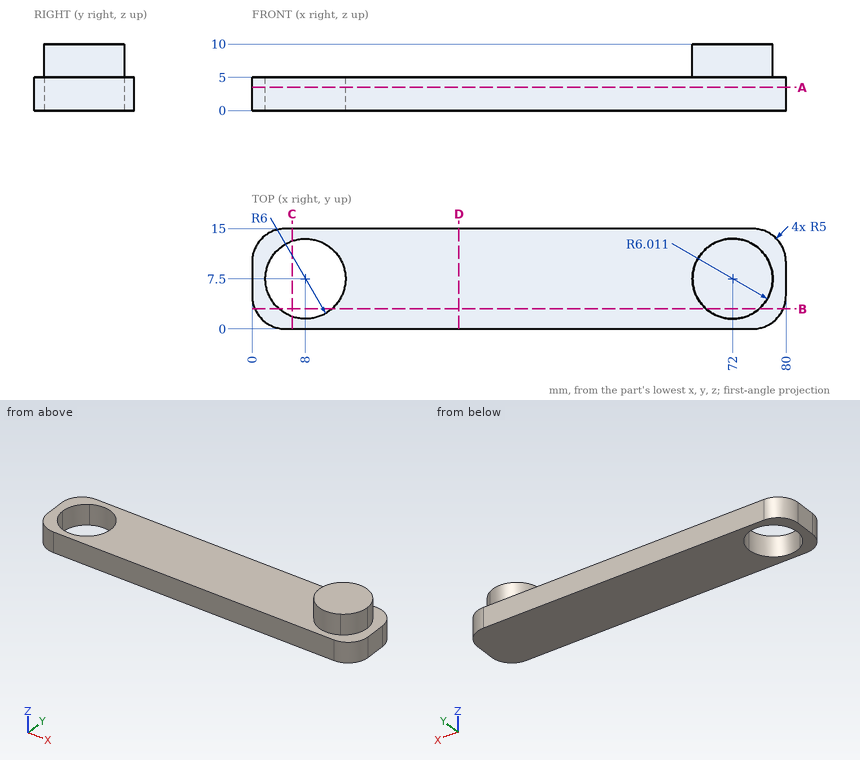
Study the drawing (mm; zero at the part's minimum x, y, z) and answer. Round coordinates to 2 decimals unless told otherwise and drop trailing zeros. Order: outer loops, then holes, each group sorted by start corner. A loop starts at its lowest first (then second) coordinate and runs counter-clockwise, first axis right, second up. Notation, with made-up numbers: (-34.75, 16) -> (-12.75, 16) arc R31 ccw to (-12.75, 45) -> close; hole circle Ø5 at (50.25, 73). An arc over 180 degrees is marked (long way). Answer as CSV lines item,"result". Start each with the question number.
(1) The part is cut by section A-A (z = 3.5). Determine the outline of the cut face in (x, y), then the cut area to 3 significant figures.
(2) The part is cut by section D-D (x = 31). Determine the outline of the cut face in (y, z), then the cut area to 3 significant figures.
(3) Flat-ended cylindrical pins translate along their axes: pin 1 Ø8 at (x, y) = (19.5, 1.5) entering from +Z; pin 2 Ø4 at (y, z) = (11.5, 8.5) entering from +X; pin 3 Ø3 at (y, z) = (2.5, 3) entering from -X. Find the tip coordinate at first contact, or state that the pin passes through.
(4) Find the intervals of material crossed by probe 1 along X at (y, z) = (7.75, 1.25) (1 decimal); probe 2 along X at (y, z) = (1, 4.5); probe 3 along Z at (x, y) = (54.5, 11.5), in increasing order. Write a range as from..to.
(5) The part is cut by section C-C (x = 6). Determine the outline of the cut face in (y, z), then the cut area to 3 significant figures.
(6) The part is cut by section B-B (y = 3). Determine the outline of the cut face in (x, z) (1 decimal), then the cut area to 3 significant figures.
Evaluation:
1,outline,"(0, 5) arc R5 ccw to (5, 0) -> (75, 0) arc R5 ccw to (80, 5) -> (80, 10) arc R5 ccw to (75, 15) -> (5, 15) arc R5 ccw to (0, 10) -> close; hole circle Ø12 at (8, 7.5)"
1,area,"1,070 mm²"
2,outline,"(0, 0) -> (15, 0) -> (15, 5) -> (0, 5) -> close"
2,area,"75.0 mm²"
3,pin 1,"z = 5"
3,pin 2,"x = 77.67"
3,pin 3,"x = 0.1"
4,probe 1,"0..2, 14..80"
4,probe 2,"2..78"
4,probe 3,"0..5"
5,outline,"(0, 0) -> (1.84, 0) -> (1.84, 5) -> (0, 5) -> close; (13.16, 0) -> (15, 0) -> (15, 5) -> (13.16, 5) -> close"
5,area,"18.4 mm²"
6,outline,"(0.4, 0) -> (4, 0) -> (4, 5) -> (0.4, 5) -> close; (12, 0) -> (79.6, 0) -> (79.6, 5) -> (76, 5) -> (76, 10) -> (68, 10) -> (68, 5) -> (12, 5) -> close"
6,area,"396 mm²"
